Geometry check sheet. Reference: the model listing, model coordinates, mm. A direction names the side the tool comes from. Give positions to 0.01 mm unless a question says otherwise; leave off trailing zeros. Write each loop counter-clockwise with the first axis right and the second up, starting at its lowest first coordinate (ties: lowest second). Pieces come first, ordered by that corner, then holes. Notation, with made-up numbers: (64, 45) - (86, 45) arc R8 ccw to (86, 58) - close; hole circle Ø10 at (7, 19). An arc over 180 degrees is marked (long way). One line per question, with ' | ' between items. Start each with the question number.
Q1. Thickness scan on L1, parallel to Y at x = 56, z = 4.25; L2, parallel to Y at x = 0, z = 0.3; L3, parallel to Z at x = 61.5, y = 3.5. Record the ranges inside material, lowest first. Write a range as [from, to].
Q2. Release check for a two-part mould opening along Y. For faces 1 (the face through (-3.7, 3.8, 3.9)), 2 (the face through (34.5, 6.5, 7.85)), 3 (the face through (5.58, 5.556, 0.394)) record: +Y half, -Y half, draft (parallel to the pull), parting line (faces both ways), or undercut.
Q3. Gauge pin test, flat ends, axial feed: P1, Ø3, axis at x = 33, y = 3.5, coming from the -Z side; P2, Ø1.5, axis at y = 2, z = 4.5, coming from the +X side. Record the tip position at first contact, or that the pin passes through.
Q4. Section check A-A on x = 8. Record the boundary of the cut face in (y, z).
Q5. Set-up check for faces 4 (the face through (5.75, 5.76, 7.46)), 5 (the face through (-0.52, 1.357, 3.881)), 6 (the face through (50, 2, 0.8)): record each of +Z, -Z, +X, -X, +Y, -Y from which the full face is reachable in a straight line by a thin tool's end or side.
Q6. Section check B-B on z = 1.5. Count the separate pieces of the cut face and the enclosed holes in it, and give its area (3 significant figures).
```python
from build123d import *

# Parameters (mm, degrees)
F0_R     = 2.4
F1_DEPTH = 7.85
F2_R     = 3.05
F3_DEPTH = 0.8
F4_R     = 3.05
F5_DEPTH = 0.8


with BuildPart() as f1:
    # F0 (on Top) → F1 (new body)
    with BuildSketch(Plane.XY):
        with BuildLine():
            ThreePointArc((0, 7.4), (-3.7, 3.7), (0, 0))
            Line((0, 0), (64, 0))
            ThreePointArc((64, 0), (67.7, 3.7), (64, 7.4))
            Line((64, 7.4), (0, 7.4))
        make_face()
        with Locations((0, 3.7)):
            Circle(F0_R, mode=Mode.SUBTRACT)
        with Locations((8, 3.7)):
            Circle(F0_R, mode=Mode.SUBTRACT)
        with Locations((16, 3.7)):
            Circle(F0_R, mode=Mode.SUBTRACT)
        with Locations((24, 3.7)):
            Circle(F0_R, mode=Mode.SUBTRACT)
        with Locations((32, 3.7)):
            Circle(F0_R, mode=Mode.SUBTRACT)
        with Locations((40, 3.7)):
            Circle(F0_R, mode=Mode.SUBTRACT)
        with Locations((48, 3.7)):
            Circle(F0_R, mode=Mode.SUBTRACT)
        with Locations((56, 3.7)):
            Circle(F0_R, mode=Mode.SUBTRACT)
        with Locations((64, 3.7)):
            Circle(F0_R, mode=Mode.SUBTRACT)
    extrude(amount=F1_DEPTH)

    # F2 (on face) → F3 (cut)
    with BuildSketch(Plane.XY.offset(7.85)):
        with Locations((0, 3.7)):
            Circle(F2_R)
        with Locations((8, 3.7)):
            Circle(F2_R)
        with Locations((16, 3.7)):
            Circle(F2_R)
        with Locations((24, 3.7)):
            Circle(F2_R)
        with Locations((32, 3.7)):
            Circle(F2_R)
        with Locations((40, 3.7)):
            Circle(F2_R)
        with Locations((48, 3.7)):
            Circle(F2_R)
        with Locations((56, 3.7)):
            Circle(F2_R)
        with Locations((64, 3.7)):
            Circle(F2_R)
    extrude(amount=-F3_DEPTH, mode=Mode.SUBTRACT)

    # F4 (on face) → F5 (cut)
    with BuildSketch(Plane(origin=(0, 0, 0), x_dir=(1, 0, 0), z_dir=(0, 0, -1))):
        with Locations((0, -3.7)):
            Circle(F4_R)
        with Locations((8, -3.7)):
            Circle(F4_R)
        with Locations((16, -3.7)):
            Circle(F4_R)
        with Locations((24, -3.7)):
            Circle(F4_R)
        with Locations((32, -3.7)):
            Circle(F4_R)
        with Locations((64, -3.7)):
            Circle(F4_R)
        with Locations((56, -3.7)):
            Circle(F4_R)
        with Locations((40, -3.7)):
            Circle(F4_R)
        with Locations((48, -3.7)):
            Circle(F4_R)
    extrude(amount=-F5_DEPTH, mode=Mode.SUBTRACT)


solid = f1.part
```
Working result:
1) L1: y = [0, 1.3], [6.1, 7.4] | L2: y = [0, 0.65], [6.75, 7.4] | L3: z = [0.8, 7.05]
2) face 1: parting line | face 2: draft | face 3: undercut
3) P1: stops at z = 0.8 | P2: stops at x = 67.58
4) outline: (0, 0) - (0.65, 0) - (0.65, 0.8) - (1.3, 0.8) - (1.3, 7.05) - (0.65, 7.05) - (0.65, 7.85) - (0, 7.85) - close; (6.1, 0.8) - (6.75, 0.8) - (6.75, 0) - (7.4, 0) - (7.4, 7.85) - (6.75, 7.85) - (6.75, 7.05) - (6.1, 7.05) - close
5) face 4: +Z | face 5: +Z, -Z | face 6: -Z
6) separate pieces: 1 | enclosed holes: 9 | area: 354 mm2
